Could you check a few things on this drawing? It's one solid part, dimensions in mm from its lowest x, y, z. A direction names the side the tool comes from. Give positions to 0.01 mm unless a question says otherwise; leave off trailing zeros. Loops run counter-clockwise (first coordinate to the right, second up) from the corner with the lowest first, then second, coordinate; pieces in that order, holes last. Notation, with made-up numbers: M 15.25,45 L 58.25,45 A9 ccw 58.25,56 Z; hole C 40,72 d5. An arc over 180 degrees is marked long. Answer in a Markdown table with one row per item. Add a question column.
1. If we section it at C-C on y = 42: List the corners of the cut face in (x, z) for me, then the cut area to 3 significant figures.
2. If we section it at D-D on x = 6.5: List the corners of the cut face in (y, z) for me, then the cut area to 4 significant figures.
3. Thinking about a two-plate mould opening in Y: for the marked faces 1, 2 and 3, which applies, released by +Y, released by -Y, zero draft, split by the parting line, or undercut?
4. Which directions (+Z, -Z, +X, -X, +Y, -Y) give clear straight access to the entire face, cutting with the end or side of a thin tool? Please do the marked faces 4, 5 and 6.
5. I'm going to push flat-ended pins straight in: pin 1 Ø4 at (y, z) = (36, 30.5) entering from +X; pin 2 Ø2.5 at (x, y) = (1.5, 8.5) entering from +Z; pin 3 Ø10 at (x, z) = (5, 27) entering from +Y. Where does each tip first touch, or does it pass through?
6. If we section it at B-B on z = 16: List the corners of the cut face in (x, y) for me.
7. I need wall thicknesses on line 1 along Y through (x, z) = (24.5, 9); line 2 along X through (y, z) = (38, 4); line 3 along Y through (x, z) = (23.5, 15.5). Which ranges of each line are inside material? Lowest first, please. Write a range as from..to.
8. If we section it at A-A on x = 31.5: List the corners of the cut face in (y, z) for me.
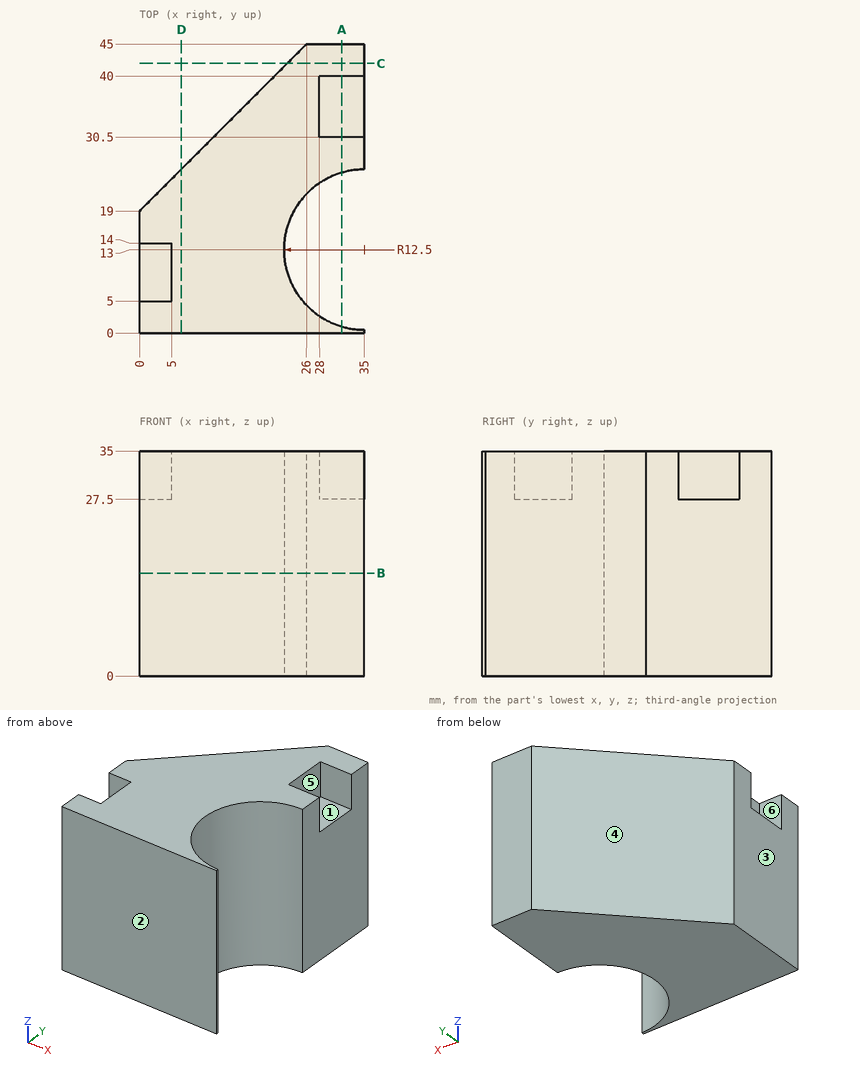
Results:
| question | item | result |
|---|---|---|
| 1 | outline | M 23,0 L 35,0 L 35,35 L 23,35 Z |
| 1 | area | 420 mm2 |
| 2 | outline | M 0,0 L 25.5,0 L 25.5,35 L 0,35 Z |
| 2 | area | 892.5 mm2 |
| 3 | face 1 | undercut |
| 3 | face 2 | released by -Y |
| 3 | face 3 | zero draft |
| 4 | face 4 | +Z, -Z, -X, +Y |
| 4 | face 5 | +Z, +X |
| 4 | face 6 | +Z, -X |
| 5 | pin 1 | x = 28 |
| 5 | pin 2 | z = 27.5 |
| 5 | pin 3 | y = 29 |
| 6 | outline | M 0,0 L 35,0 L 35,0.5 A12.5 cw 35,25.5 L 35,45 L 26,45 L 0,19 Z |
| 7 | line 1 | 0..6.22, 19.78..43.5 |
| 7 | line 2 | 19..35 |
| 7 | line 3 | 0..8.1, 17.9..42.5 |
| 8 | outline | M 0,0 L 1,0 L 1,35 L 0,35 Z; M 25,0 L 45,0 L 45,35 L 40,35 L 40,27.5 L 30.5,27.5 L 30.5,35 L 25,35 Z |
